```python
from build123d import *

# Parameters (mm, degrees)
BOSS_EXTRUDE2_DEPTH = 331.382
SKETCH3_W           = 66
SKETCH3_H           = 122
CUT_EXTRUDE2_DEPTH  = 128.0000001
SKETCH4_W           = 240
SKETCH4_H           = 111.6
CUT_EXTRUDE3_DEPTH  = 332.3820001
SKETCH5_W           = 254
SKETCH5_H           = 35.4
BOSS_EXTRUDE3_DEPTH = 331.382


with BuildPart() as part:
    # Sketch2 → Boss-Extrude2 (new body)
    with BuildSketch(Plane.XY):
        with BuildLine():
            Line((-127, 127), (127, 127))
            add(Edge.make_bspline(
                [(-127, 127), (0, -127), (127, 127)],
                knots=[0.056028396, 0.056028396, 0.056028396, 0.943971604, 0.943971604, 0.943971604], degree=2))
        make_face()
    extrude(amount=BOSS_EXTRUDE2_DEPTH)

    # Sketch3 → Cut-Extrude2 (cut, through all)
    with BuildSketch(Plane(origin=(0, 127, 0), x_dir=(1, 0, 0), z_dir=(0, 1, 0))):
        with Locations((0, -82.8455)):
            Rectangle(SKETCH3_W, SKETCH3_H)
        with Locations((0, -248.5365)):
            Rectangle(SKETCH3_W, SKETCH3_H)
    extrude(amount=-CUT_EXTRUDE2_DEPTH, mode=Mode.SUBTRACT)

    # Sketch4 → Cut-Extrude3 (cut, through all)
    with BuildSketch(Plane(origin=(0, 0, 0), x_dir=(-1, 0, 0), z_dir=(0, 0, -1))):
        with Locations((0, 55.8)):
            Rectangle(SKETCH4_W, SKETCH4_H)
    extrude(amount=-CUT_EXTRUDE3_DEPTH, mode=Mode.SUBTRACT)

    # Sketch5 → Boss-Extrude3 (add)
    with BuildSketch(Plane.XY.offset(331.382)):
        with Locations((0, 144.7)):
            Rectangle(SKETCH5_W, SKETCH5_H)
    extrude(amount=-BOSS_EXTRUDE3_DEPTH)


solid = part.part
```
The listing builds one solid part. Answer for the finished solid, in the listing's coordinates (mm). A direction names the side the tool comes from. Give positions to 0.01 mm unless a question says otherwise; leave off trailing zeros. Loops run counter-clockwise (first coordinate to the right, second up) from the corner with the lowest first, then second, coordinate; pieces in that order, holes last. Notation, with made-up numbers: M -12,16 L 0,16 A17 ccw 0,42 Z; hole C 65,50.25 d9. An arc over 180 degrees is marked long. One line per item, written item: value.
Q1. For faces 1 (the face through (-2, 137, 0)), 2 (the face through (0, 127, 249)), determine the directions among +Z, -Z, +X, -X, +Y, -Y from which every point of the face is accessible in a straight line to the end or side of a thin tool.
Working result:
face 1: -Z, +X, -X, +Y, -Y
face 2: -Y
Q2. Determine the mould class of faces 3 (the face through (0, 119, 187.536)), 4 (the face through (0, 119, 309.536)), 5 (the face through (-2, 137, 331.382)), 6 (the face through (127, 144, 168)) for opening direction Z: +Z half, -Z half, draft (parallel to the pull), parting line (faces both ways), or undercut.
Working result:
face 3: undercut
face 4: undercut
face 5: +Z half
face 6: draft
Q3. A cutting plane is placed at A-A on x = -1. Determine the outline of the cut face in (y, z).
Working result:
outline: M 111.6,0 L 162.4,0 L 162.4,331.38 L 111.6,331.38 L 111.6,309.54 L 127,309.54 L 127,187.54 L 111.6,187.54 L 111.6,143.85 L 127,143.85 L 127,21.85 L 111.6,21.85 Z
Q4. Find the intervals of material crossed by line 1 (Z direction, x = 27.5, y = 126.5); line 2 (Y direction, x = -5.5, z = 43); line 3 (X direction, y = 126, z = 109.5), in increasing order. Write a range as from..to.
Working result:
line 1: z = 0..21.85, 143.85..187.54, 309.54..331.38
line 2: y = 127..162.4
line 3: x = -126.5..-33, 33..126.5
Q5. Flat-ended cylindrical pins translate along their axes: P1, Ø1.5, axis at y = 118.5, z = 269.5, coming from the -X side; P2, Ø12.5, axis at y = 119, z = 271, coming from the +X side; P3, Ø12.5, axis at y = 116, z = 96.5, coming from the -X side. Find the tip coordinate at first contact, or state that the pin passes through.
Working result:
P1: stops at x = -123.06
P2: stops at x = 126.12
P3: stops at x = -124.6
